```python
from build123d import *

# Parameters (mm, degrees)
F0_W     = 340
F0_H     = 500
F0_W_2   = 300
F0_H_2   = 20
F1_DEPTH = 10
F2_DEPTH = 35


# Not quite as in the source:
# - a feature names something its author has since deleted; it is built from what else it names


with BuildPart() as f1:
    # F0 (on Front) → F1 (new body)
    with BuildSketch(Plane.XZ):
        with Locations((-54.2285538465, 60.7086803179)):
            Rectangle(F0_W, F0_H)
        with Locations((-54.2285538465, -129.2913196821)):
            Rectangle(F0_W_2, F0_H_2, mode=Mode.SUBTRACT)
        with Locations((-54.2285538465, -29.2913196821)):
            Rectangle(F0_W_2, F0_H_2, mode=Mode.SUBTRACT)
        with Locations((-54.2285538465, 70.7086803179)):
            Rectangle(F0_W_2, F0_H_2, mode=Mode.SUBTRACT)
    extrude(amount=F1_DEPTH)

    # F0 (on Front) → F2 (join)
    with BuildSketch(Plane.XZ):
        with Locations((-54.2285538465, 70.7086803179)):
            Rectangle(F0_W_2, F0_H_2)
        with Locations((-54.2285538465, -29.2913196821)):
            Rectangle(F0_W_2, F0_H_2)
        with Locations((-54.2285538465, -129.2913196821)):
            Rectangle(F0_W_2, F0_H_2)
    extrude(amount=F2_DEPTH)


solid = f1.part
```
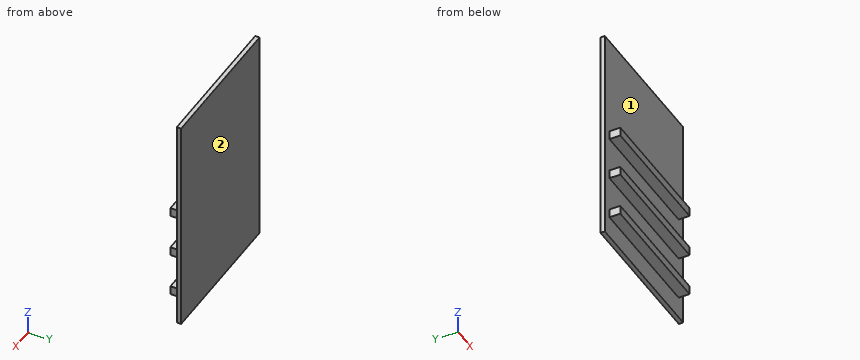
The listing builds one solid part. Answer for the finished solid, in the listing's coordinates (mm). Face numbers are marked on the shaded views. Round coordinates to 2 decimals unless told otherwise and drop trailing zeros. Loops run counter-clockwise (first coordinate to the right, second up) from the corner with the lowest first, then second, coordinate; pieces in that order, holes last. Notation, with made-up numbers: (67.5, 44) - (115.5, 44) arc R20 cw to (115.5, 83) - close; hole circle Ø10 at (44.25, -22.75). An arc over 180 degrees is marked (long way). Return JSON: item names as keys, results as strings. Group by question number.
1. The part is cut by section A-A on x = -116.5. Determine the outline of the cut face in (y, z), then the cut area to 3 significant figures.
2. Each of these flat-tipped pins is pushed along its axis until it touches: P1, Ø3, axis at x = -149.5, y = -18, coming from the -Z side; P2, Ø6, axis at x = -173, z = -102.5, coming from the +Y side; P3, Ø2, axis at x = -18.5, z = 7, coming from the -Y side; P4, Ø16, axis at y = -25.5, z = -31.5, coming from the -X side. Where does it stop, or does it pass through?
3. Consider probe 1 along Z at (x, y) = (68, -21.5); probe 2 along Y at (x, z) = (-24.5, 184.5). Determine where each line is inside the solid, lowest interval first.
4. The part is cut by section C-C on z = -30. Determine the outline of the cut face in (x, y).
5. The part is cut by section D-D on z = 237. Determine the outline of the cut face in (x, y), then the cut area to 3 significant figures.
6. The part is cut by section B-B on y = -19. Determine the outline of the cut face in (x, z), then the cut area to 3 significant figures.
7. The mould has two halves that part along Z. Classify the marked faces 1 and 2: pulls with the +Z half, pulls with the -Z half, needs draft (parallel to the pull), parting line crosses it, or undercut.
Resolved:
{
 "1": {"outline": "(-35, -139.29) - (-10, -139.29) - (-10, -189.29) - (0, -189.29) - (0, 310.71) - (-10, 310.71) - (-10, 80.71) - (-35, 80.71) - (-35, 60.71) - (-10, 60.71) - (-10, -19.29) - (-35, -19.29) - (-35, -39.29) - (-10, -39.29) - (-10, -119.29) - (-35, -119.29) - close", "area": "6,500 mm²"},
 "2": {"P1": "stops at z = -139.29", "P2": "stops at y = 0", "P3": "stops at y = -10", "P4": "stops at x = -204.23"},
 "3": {"probe 1": "z = -139.29 to -119.29, -39.29 to -19.29, 60.71 to 80.71", "probe 2": "y = -10 to 0"},
 "4": {"outline": "(-224.23, -10) - (-204.23, -10) - (-204.23, -35) - (95.77, -35) - (95.77, -10) - (115.77, -10) - (115.77, 0) - (-224.23, 0) - close"},
 "5": {"outline": "(-224.23, -10) - (115.77, -10) - (115.77, 0) - (-224.23, 0) - close", "area": "3,400 mm²"},
 "6": {"outline": "(-204.23, -139.29) - (95.77, -139.29) - (95.77, -119.29) - (-204.23, -119.29) - close; (-204.23, -39.29) - (95.77, -39.29) - (95.77, -19.29) - (-204.23, -19.29) - close; (-204.23, 60.71) - (95.77, 60.71) - (95.77, 80.71) - (-204.23, 80.71) - close", "area": "18,000 mm²"},
 "7": {"face 1": "undercut", "face 2": "needs draft"}
}
